```python
from build123d import *

# Parameters (mm, degrees)
CUT_EXTRUDE_1_REACH = 285.549
SKETCH_5_R          = 10


with BuildPart() as part:
    # 草圖4 → 旋轉1 (revolve)
    with BuildSketch(Plane.XY, mode=Mode.PRIVATE) as revolve_1_sk:
        Polygon((120, 20), (120, 5), (94.5, 5), (94.5, 0), (200, 0), (200, 20), align=None)
    revolve(revolve_1_sk.sketch.rotate(Axis((0, 45.980375907, 0), (0, -1, 0)), 180), axis=Axis((0, 45.980375907, 0), (0, -1, 0)))

    # 草圖5 → 除料-伸長1 (cut, up to next)
    with BuildSketch(Plane(origin=(0, 20, 0), x_dir=(1, 0, 0), z_dir=(0, 1, 0)), mode=Mode.PRIVATE) as cut_extrude_1_sk1:
        with Locations(Location((0, 160, 0), (0, 0, 180))):
            Circle(SKETCH_5_R)
    cut_extrude_1_tool1 = extrude(cut_extrude_1_sk1.sketch, amount=-CUT_EXTRUDE_1_REACH, mode=Mode.PRIVATE) & part.part
    # 草圖5 → 除料-伸長1 (cut, up to next)
    with BuildSketch(Plane(origin=(0, 20, 0), x_dir=(1, 0, 0), z_dir=(0, 1, 0)), mode=Mode.PRIVATE) as cut_extrude_1_sk2:
        with Locations(Location((138.564064606, 80, 0), (0, 0, 180))):
            Circle(SKETCH_5_R)
    cut_extrude_1_tool2 = extrude(cut_extrude_1_sk2.sketch, amount=-CUT_EXTRUDE_1_REACH, mode=Mode.PRIVATE) & part.part
    # 草圖5 → 除料-伸長1 (cut, up to next)
    with BuildSketch(Plane(origin=(0, 20, 0), x_dir=(1, 0, 0), z_dir=(0, 1, 0)), mode=Mode.PRIVATE) as cut_extrude_1_sk3:
        with Locations(Location((138.564064606, -80, 0), (0, 0, 180))):
            Circle(SKETCH_5_R)
    cut_extrude_1_tool3 = extrude(cut_extrude_1_sk3.sketch, amount=-CUT_EXTRUDE_1_REACH, mode=Mode.PRIVATE) & part.part
    # 草圖5 → 除料-伸長1 (cut, up to next)
    with BuildSketch(Plane(origin=(0, 20, 0), x_dir=(1, 0, 0), z_dir=(0, 1, 0)), mode=Mode.PRIVATE) as cut_extrude_1_sk4:
        with Locations(Location((0, -160, 0), (0, 0, 180))):
            Circle(SKETCH_5_R)
    cut_extrude_1_tool4 = extrude(cut_extrude_1_sk4.sketch, amount=-CUT_EXTRUDE_1_REACH, mode=Mode.PRIVATE) & part.part
    # 草圖5 → 除料-伸長1 (cut, up to next)
    with BuildSketch(Plane(origin=(0, 20, 0), x_dir=(1, 0, 0), z_dir=(0, 1, 0)), mode=Mode.PRIVATE) as cut_extrude_1_sk5:
        with Locations(Location((-138.564064605, -80, 0), (0, 0, 180))):
            Circle(SKETCH_5_R)
    cut_extrude_1_tool5 = extrude(cut_extrude_1_sk5.sketch, amount=-CUT_EXTRUDE_1_REACH, mode=Mode.PRIVATE) & part.part
    # 草圖5 → 除料-伸長1 (cut, up to next)
    with BuildSketch(Plane(origin=(0, 20, 0), x_dir=(1, 0, 0), z_dir=(0, 1, 0)), mode=Mode.PRIVATE) as cut_extrude_1_sk6:
        with Locations(Location((-138.564064606, 80, 0), (0, 0, 180))):
            Circle(SKETCH_5_R)
    cut_extrude_1_tool6 = extrude(cut_extrude_1_sk6.sketch, amount=-CUT_EXTRUDE_1_REACH, mode=Mode.PRIVATE) & part.part
    add(cut_extrude_1_tool1.solids().sort_by_distance((0, 20, -160))[0], mode=Mode.SUBTRACT)
    add(cut_extrude_1_tool2.solids().sort_by_distance((138.564065, 20, -80))[0], mode=Mode.SUBTRACT)
    add(cut_extrude_1_tool3.solids().sort_by_distance((138.564065, 20, 80))[0], mode=Mode.SUBTRACT)
    add(cut_extrude_1_tool4.solids().sort_by_distance((0, 20, 160))[0], mode=Mode.SUBTRACT)
    add(cut_extrude_1_tool5.solids().sort_by_distance((-138.564065, 20, 80))[0], mode=Mode.SUBTRACT)
    add(cut_extrude_1_tool6.solids().sort_by_distance((-138.564065, 20, -80))[0], mode=Mode.SUBTRACT)


solid = part.part
```
CAD build for the part. Positions are in the model's coordinates, mm. A direction names the side the tool comes from. Round coordinates to 2 decimals unless told otherwise and drop trailing zeros. Order: outer loops, then holes, each group sorted by start corner. A loop starts at its lowest first (then second) coordinate and runs counter-clockwise, first axis right, second up. Notation, with made-up numbers: (68, 40) - (104, 40) arc R27 cw to (104, 65) - close; hole circle Ø5 at (9, 64). An arc over 180 degrees is marked (long way). Answer in a Markdown table with one row per item. Add a question column.
(1) Drop flat-ended pins along their axis: pin 1 Ø12 at (x, y) = (-151, 12.5) entering from -Z; pin 2 Ø4 at (x, y) = (50.5, 9) entering from +Z; pin 3 Ø4 at (x, y) = (74.5, 8.5) entering from +Z; pin 4 Ø12 at (x, z) = (138.56, 80) entering from +Y. Give the stop position or say it passes through.
(2) Band-saw the part on D-D on z = 80. List the corners of the cut face in (x, y).
(3) 3-axis set-ups, long thin cutter, end or side, ignore diameter. For faces 1 (the face through (-35, 5, 88)), 2 (the face through (-131.194, 10.14, 86.758)): which of +Z, -Z, +X, -X, +Y, -Y reach the whole face in a straight line?
(4) Mould opens along Z. For faces 3 (the face through (-86, 20, 86)), 4 (the face through (-190.764, 10.14, -60.075)), 5 (the face through (-64.511, 12.395, -101.184)) say: +Z half, -Z half, draft (parallel to the pull), parting line (faces both ways), or undercut.
(5) Band-saw the part on B-B on y = 8. List the corners of the cut face in (x, z).
(6) Band-saw the part on C-C on z = 0. List the corners of the cut face in (x, y), and give its area (4 significant figures).
(7) Probe L1, parallel to Z at x = 0, y = 3.65; L2, parallel to Z at x = 0, y = 16.5; L3, parallel to X at y = 6.5, z = -77. List the from-to ranges inside material, lowest first. Write a range as [from, to].
(8) Band-saw the part on A-A on x = 0. List the corners of the cut face in (y, z), and give its area (4 significant figures).
Data:
| question | item | result |
|---|---|---|
| 1 | pin 1 | stops at z = -137.75 |
| 1 | pin 2 | stops at z = 194.03 |
| 1 | pin 3 | stops at z = 186.4 |
| 1 | pin 4 | passes through |
| 2 | outline | (-183.3, 0) - (-148.56, 0) - (-148.56, 20) - (-183.3, 20) - close; (-128.56, 0) - (-50.3, 0) - (-50.3, 5) - (-89.44, 5) - (-89.44, 20) - (-128.56, 20) - close; (50.3, 0) - (128.56, 0) - (128.56, 20) - (89.44, 20) - (89.44, 5) - (50.3, 5) - close; (148.56, 0) - (183.3, 0) - (183.3, 20) - (148.56, 20) - close |
| 3 | face 1 | +Y |
| 3 | face 2 | +Y, -Y |
| 4 | face 3 | draft |
| 4 | face 4 | parting line |
| 4 | face 5 | undercut |
| 5 | outline | circle Ø400 at (0, 0); hole circle Ø20 at (-138.56, -80); hole circle Ø20 at (-138.56, 80); hole circle Ø240 at (0, 0); hole circle Ø20 at (0, -160); hole circle Ø20 at (0, 160); hole circle Ø20 at (138.56, -80); hole circle Ø20 at (138.56, 80) |
| 6 | outline | (-200, 0) - (-94.5, 0) - (-94.5, 5) - (-120, 5) - (-120, 20) - (-200, 20) - close; (94.5, 0) - (200, 0) - (200, 20) - (120, 20) - (120, 5) - (94.5, 5) - close |
| 6 | area | 3,455 mm^2 |
| 7 | L1 | z = [-200, -170], [-150, -94.5], [94.5, 150], [170, 200] |
| 7 | L2 | z = [-200, -170], [-150, -120], [120, 150], [170, 200] |
| 7 | L3 | x = [-184.58, -148.1], [-129.02, -92.04], [92.04, 129.02], [148.1, 184.58] |
| 8 | outline | (0, -200) - (20, -200) - (20, -170) - (0, -170) - close; (0, -150) - (20, -150) - (20, -120) - (5, -120) - (5, -94.5) - (0, -94.5) - close; (0, 94.5) - (5, 94.5) - (5, 120) - (20, 120) - (20, 150) - (0, 150) - close; (0, 170) - (20, 170) - (20, 200) - (0, 200) - close |
| 8 | area | 2,655 mm^2 |
